Check sheet for the modelled part. Datum: model origin and axes. Units: mm. A direction names the side the tool comes from. Round coordinates to 2 decimals unless told otherwise and drop trailing zeros. Order: outer loops, then holes, each group sorted by start corner. A loop starts at its lowest first (then second) coordinate and runs counter-clockwise, first axis right, second up.
Q1. Cross-section at C-C on x = 0. Give the number of separate pieces and of enclosed holes in the cut face, then the cut area to 3 significant figures.
Q2. Depth check by flat-ended pin: P1, Ø5.5, axis at x = 0, z = -113, coming from the -Y side; P2, Ø2, axis at x = 0, z = -113, coming from the -Y side. Enter the tip coordinate at first touch or a pass-through.
Q3. Cross-section at B-B on y = -24. Record the cut outline in (x, z).
Q4. Set-up check for faces 4 (the cylindrical face through (1.014, -27.014, -83.436)), 5 (the cylindrical face through (-1.35, -22.96, -186.97)): record each of +Z, -Z, +X, -X, +Y, -Y from which the full face is reachable in a straight line by a thin tool's end or side.
Q5. Scan lines: probe 1 along X at (y, z) = (-22.6, -63); probe 2 along Y at (x, z) = (5.5, -121.5); probe 3 along Y at (x, z) = (-1.25, -65). Record each from-to range of solid material in increasing order.
Q6. Cross-section at A-A on z = -163. Record the cut outline in (x, y).
Q7. Cross-section at D-D on z = -145.5. Record the cut outline in (x, y), then the cut area to 3 significant figures.
Q8. Mould release check, pull along X, two halves, no side actions. Record for faces 1 (the flat face through (-2, -26, -138)), 2 (the flat face through (0, -28, -124)), 3 (the flat face through (-6, -23, -124)): +X half, -X half, draft (parallel to the pull), parting line (faces both ways), or undercut.
from build123d import *

# Parameters (mm, degrees)
BOSS_EXTRUDE1_START                          = -50
SKETCH1_W                                    = 12
SKETCH1_H                                    = 8
BOSS_EXTRUDE1_DEPTH                          = 150
CUT_EXTRUDE1_REACH                           = 154.709
SKETCH2_R                                    = 0.75
CBORE_FOR_M3_HEX_HEAD_CAP_SCREW1_D           = 3.4
CBORE_FOR_M3_HEX_HEAD_CAP_SCREW1_CBORE_D     = 9.351
CBORE_FOR_M3_HEX_HEAD_CAP_SCREW1_CBORE_DEPTH = 2
LPATTERN2_COUNT                              = 6
LPATTERN2_PITCH                              = 25


with BuildPart() as part:
    # Sketch1 → Boss-Extrude1 (new body)
    with BuildSketch(Plane.XY.offset(BOSS_EXTRUDE1_START)):
        with Locations((0, -24)):
            Rectangle(SKETCH1_W, SKETCH1_H)
    extrude(amount=-BOSS_EXTRUDE1_DEPTH)

    # Sketch2 → Cut-Extrude1 (cut, up to next)
    with BuildSketch(Plane.XY.offset(-50), mode=Mode.PRIVATE) as cut_extrude1_sk1:
        with Locations((-6, -26)):
            Circle(SKETCH2_R)
    cut_extrude1_tool1 = extrude(cut_extrude1_sk1.sketch, amount=-CUT_EXTRUDE1_REACH, mode=Mode.PRIVATE) & part.part
    # Sketch2 → Cut-Extrude1 (cut, up to next)
    with BuildSketch(Plane.XY.offset(-50), mode=Mode.PRIVATE) as cut_extrude1_sk2:
        with Locations((6, -26)):
            Circle(SKETCH2_R)
    cut_extrude1_tool2 = extrude(cut_extrude1_sk2.sketch, amount=-CUT_EXTRUDE1_REACH, mode=Mode.PRIVATE) & part.part
    add(cut_extrude1_tool1.solids().sort_by_distance((-6, -26, -50))[0], mode=Mode.SUBTRACT)
    add(cut_extrude1_tool2.solids().sort_by_distance((6, -26, -50))[0], mode=Mode.SUBTRACT)

    # CBORE for M3 Hex Head Cap Screw1 (through all)
    with Locations(Plane(origin=(0, -28, 0), x_dir=(-1, 0, 0), z_dir=(0, -1, 0))):
        with Locations((0, 63)):
            cbore_for_m3_hex_head_cap_screw1 = CounterBoreHole(CBORE_FOR_M3_HEX_HEAD_CAP_SCREW1_D / 2, CBORE_FOR_M3_HEX_HEAD_CAP_SCREW1_CBORE_D / 2, CBORE_FOR_M3_HEX_HEAD_CAP_SCREW1_CBORE_DEPTH)

    # LPattern2: CBORE for M3 Hex Head Cap Screw1 ×6
    with Locations(*[(0, 0, -i * LPATTERN2_PITCH) for i in range(1, LPATTERN2_COUNT)]):
        add(cbore_for_m3_hex_head_cap_screw1, mode=Mode.SUBTRACT)


solid = part.part
Results found:
1. separate pieces: 7
1. enclosed holes: 0
1. area: 965 mm2
2. P1: stops at y = -26
2. P2: passes through
3. outline: (-6, -200) - (6, -200) - (6, -50) - (-6, -50) - close; hole circle Ø3.4 at (0, -188); hole circle Ø3.4 at (0, -163); hole circle Ø3.4 at (0, -138); hole circle Ø3.4 at (0, -113); hole circle Ø3.4 at (0, -88); hole circle Ø3.4 at (0, -63)
4. face 4: -Y
4. face 5: +Y, -Y
5. probe 1: x = -6 to -1.7, 1.7 to 6
5. probe 2: y = -28 to -26.56, -25.44 to -20
5. probe 3: y = -26 to -20
6. outline: (-6, -28) - (-4.68, -28) - (-4.68, -26) - (-1.7, -26) - (-1.7, -20) - (-6, -20) - (-6, -25.25) arc R0.75 cw to (-6, -26.75) - close; (1.7, -26) - (4.68, -26) - (4.68, -28) - (6, -28) - (6, -26.75) arc R0.75 cw to (6, -25.25) - (6, -20) - (1.7, -20) - close
7. outline: (-6, -28) - (6, -28) - (6, -26.75) arc R0.75 cw to (6, -25.25) - (6, -20) - (-6, -20) - (-6, -25.25) arc R0.75 cw to (-6, -26.75) - close
7. area: 94.2 mm2
8. face 1: undercut
8. face 2: draft
8. face 3: -X half
